CAD build for the part. Positions are in the model's coordinates, mm. Face numbers are marked on the shaded views. A direction names the side the tool comes from. Give positions to 0.01 mm unless a question says otherwise; leave off trailing zeros. Write each loop counter-clockwise with the first axis right and the second up, starting at its lowest first coordinate (ties: lowest second). Pieces come first, ordered by that corner, then holes. Notation, with made-up numbers: (50, 25) - (69, 25) arc R25 ccw to (69, 54) - close; hole circle Ø5 at (81.25, -6). An arc over 180 degrees is marked (long way). Write item = value, one per line. Start each with the question number.
Autodesk Inventor part; units mm, degrees
ref_plane "YZ Plane" through (0, 0, 0) normal (1, 0, 0) x (0, 1, 0)
ref_plane "XZ Plane" through (0, 0, 0) normal (0, 1, 0) x (-1, 0, 0)
ref_plane "XY Plane" through (0, 0, 0) normal (0, 0, 1) x (1, 0, 0)
sketch "Sketch1" plane through (0, 0, 0) normal (0, 1, 0) x (-1, 0, 0)
  line L0 (-25, -10) -> (25, -10)
  line L1 (25, -10) -> (25, 10)
  line L2 (25, 10) -> (-25, 10)
  line L3 (-25, 10) -> (-25, -10)
  line L4 (-25, 0) -> (25, 0) construction
  line L5 (0, -10) -> (0, 10) construction
  point P0 (0, 0)
  point P1 (0, 0)
  dimension "d0" = 50
  dimension "d1" = 20
extrude "Extrusion1" add sketch "Sketch1" along normal blind 2
sketch "Sketch2" plane through (0, 2, 0) normal (0, 1, 0) x (1, 0, 0)
  line L0 (25, -10) -> (25, 10) construction
  line L1 (25, 0) -> (-30.0792, 0) construction
  line L2 (25, 10) -> (-25, 10) construction
  line L3 (0, 10) -> (0, -10) construction
  line L4 (-25, -10) -> (25, -10) construction
  circle A0 centre (18.5, 0) radius 1.5
  circle A1 centre (-18.5, 0) radius 1.5
  point P0 (0, 0)
  dimension "d4" = 3
  dimension "d5" = 37
extrude "Extrusion2" cut sketch "Sketch2" against normal blind 2
sketch "Sketch6" plane through (0, 2, 0) normal (0, 1, 0) x (1, 0, 0)
  line L0 (25, 10) -> (-25, 10) construction
  line L1 (0, 10) -> (0, -10) construction
  line L2 (-25, -10) -> (25, -10) construction
  line L3 (6.5, 10) -> (13.5, 10)
  line L4 (13.5, 10) -> (13.5, -10)
  line L5 (13.5, -10) -> (6.5, -10)
  line L6 (6.5, -10) -> (6.5, 10)
  line L7 (-6.5, 10) -> (-13.5, 10)
  line L8 (-13.5, 10) -> (-13.5, -10)
  line L9 (-13.5, -10) -> (-6.5, -10)
  line L10 (-6.5, -10) -> (-6.5, 10)
  point P0 (0, 0)
  dimension "d19" = 7
  dimension "d20" = 6.5
extrude "Extrusion5" add sketch "Sketch6" along normal blind 50
sketch "Sketch7" plane through (0, 52, 0) normal (0, 1, 0) x (1, 0, 0)
  line L0 (6.5, 10) -> (-6.5, 10) construction
  line L1 (0, 10) -> (0, -10) construction
  line L2 (-6.5, -10) -> (6.5, -10) construction
  circle A0 centre (10, 0) radius 1.75
  line L3 (13.5, -10) -> (13.5, 10) construction
  circle A1 centre (-10, 0) radius 1.75
  point P0 (0, 0)
  dimension "d23" = 3.5
  dimension "d24" = 3.5
extrude "Extrusion6" cut sketch "Sketch7" against normal blind 6
properties part number "ir_sensor_support"
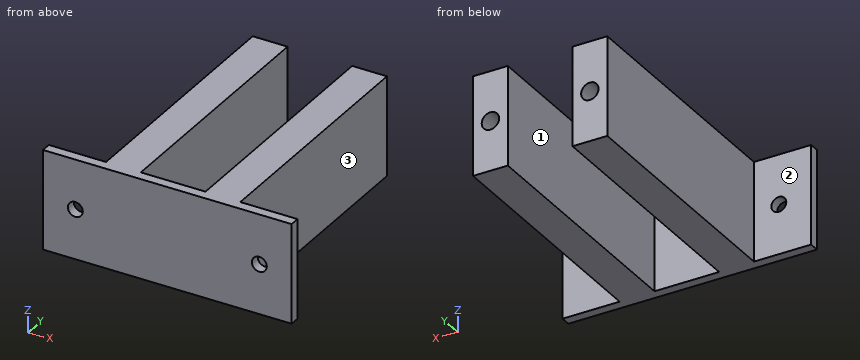
1. Pin check, flat tips, straight feed: pin 1 Ø1.8 at (x, z) = (-10.5, 0) entering from +Y; pin 2 Ø6 at (y, z) = (25, 4.5) entering from -X; pin 3 Ø5 at (x, y) = (2.5, 29) entering from -Z; pin 4 Ø9 at (x, z) = (-21, 3.5) entering from +Y. Stop position of each tip, or through.
2. Cut at D-D (z = 6). Give the cut face in (x, y).
3. Tool access for the marked faces 1, 2 and 3: list every direction of +Z, -Z, +X, -X, +Y, -Y with a clear straight run to the whole face (end or side of a thin tool).
4. Cut at A-A (z = 0). Give the cut face in (x, y).
5. Cut at C-C (x = -18.5). Give the cut face in (y, z), then the cut area to 3 significant figures.
6. Cut at B-B (y = 14). Give the cut face in (x, z), then the cut area to 3 significant figures.
7. Wall check: line 1 along X through (y, z) = (49.85, 0); line 2 along X through (y, z) = (1, 0); line 3 along Z through (x, y) = (18.5, 1.65). Give the ranges that are in metal, low to high.
Output:
q1.pin_1 = 46
q1.pin_2 = -13.5
q1.pin_3 = through
q1.pin_4 = 2
q2.outline = (-25, 0) - (25, 0) - (25, 2) - (13.5, 2) - (13.5, 52) - (6.5, 52) - (6.5, 2) - (-6.5, 2) - (-6.5, 52) - (-13.5, 52) - (-13.5, 2) - (-25, 2) - close
q3.face_1 = +Z, -Z, +Y
q3.face_2 = +Z, -Z, -X, +Y
q3.face_3 = +Z, -Z, +X, +Y
q4.outline = (-25, 0) - (-20, 0) - (-20, 2) - (-25, 2) - close; (-17, 0) - (17, 0) - (17, 2) - (13.5, 2) - (13.5, 52) - (11.75, 52) - (11.75, 46) - (8.25, 46) - (8.25, 52) - (6.5, 52) - (6.5, 2) - (-6.5, 2) - (-6.5, 52) - (-8.25, 52) - (-8.25, 46) - (-11.75, 46) - (-11.75, 52) - (-13.5, 52) - (-13.5, 2) - (-17, 2) - close; (20, 0) - (25, 0) - (25, 2) - (20, 2) - close
q5.outline = (0, -10) - (2, -10) - (2, -1.5) - (0, -1.5) - close; (0, 1.5) - (2, 1.5) - (2, 10) - (0, 10) - close
q5.area = 34.0 mm2
q6.outline = (-13.5, -10) - (-6.5, -10) - (-6.5, 10) - (-13.5, 10) - close; (6.5, -10) - (13.5, -10) - (13.5, 10) - (6.5, 10) - close
q6.area = 280 mm2
q7.line_1 = -13.5 to -11.75, -8.25 to -6.5, 6.5 to 8.25, 11.75 to 13.5
q7.line_2 = -25 to -20, -17 to 17, 20 to 25
q7.line_3 = -10 to -1.5, 1.5 to 10
